```python
from build123d import *

# Parameters (mm, degrees)
RESSALTO_EXTRUS_O1_DEPTH = 6
CORTE_EXTRUS_O1_DEPTH    = 428.242320001
FILETE1_R                = 5
RESSALTO_EXTRUS_O3_DEPTH = 7
RESSALTO_EXTRUS_O4_DEPTH = 6
FILETE2_R                = 5
ESBO_O13_W               = 15
ESBO_O13_H               = 6
CORTE_EXTRUS_O2_DEPTH    = 428.242320001
ESBO_O15_W               = 15
ESBO_O15_H               = 6
CORTE_EXTRUS_O3_DEPTH    = 428.242320001


with BuildPart() as part:
    # Esboço2 → Ressalto-extrusão1 (new body)
    with BuildSketch(Plane.XY):
        Polygon((0, 0), (0, 400), (50, 400), (150, 20), (150, 0), align=None)
    extrude(amount=RESSALTO_EXTRUS_O1_DEPTH)

    # Esboço7 → Corte-extrusão1 (cut, through all)
    with BuildSketch(Plane(origin=(0, 0, 0), x_dir=(-1, 0, 0), z_dir=(0, 0, -1))):
        Polygon((-32.276413741, 20), (-32.276413741, 310), (-120, 20), align=None)
    extrude(amount=-CORTE_EXTRUS_O1_DEPTH, mode=Mode.SUBTRACT)

    # Filete1
    filete1_edges = [part.edges().sort_by_distance(p)[0] for p in [
        (32.276413741, 20, 3),
        (120, 20, 3),
        (32.276413741, 310, 3),
    ]]
    fillet(filete1_edges, radius=FILETE1_R)

    # Esboço11 → Ressalto-extrusão3 (add)
    with BuildSketch(Plane(origin=(0, 0, 0), x_dir=(-1, 0, 0), z_dir=(0, 0, -1))):
        Polygon((-85.790275479, 133.09182096), (-32.276413741, 133.09182096), (-32.276413741, 164.53133753), (-76.279974983, 164.53133753), align=None)
    extrude(amount=-RESSALTO_EXTRUS_O3_DEPTH)

    # Esboço12 → Ressalto-extrusão4 (add)
    with BuildSketch(Plane(origin=(0, 0, 0), x_dir=(-1, 0, 0), z_dir=(0, 0, -1))):
        Polygon((-85.790275479, 133.09182096), (-32.276413741, 29.65724659), (-27.594715127, 20), (-48.670406936, 20), (-94.468741252, 104.402215557), align=None)
    extrude(amount=-RESSALTO_EXTRUS_O4_DEPTH)

    # Filete2
    filete2_edges = [part.edges().sort_by_distance(p)[0] for p in [
        (32.276413741, 133.09182096, 3),
        (32.276413741, 164.53133753, 3),
        (85.790275479, 133.09182096, 3),
        (76.279974983, 164.53133753, 3),
        (94.468741252, 104.402215557, 3),
        (32.276413741, 29.65724659, 3),
        (48.670406936, 20, 3),
    ]]
    fillet(filete2_edges, radius=FILETE2_R)

    # Esboço13 → Corte-extrusão2 (cut, through all)
    with BuildSketch(Plane.XY.offset(6)):
        with Locations((7.5, 397)):
            Rectangle(ESBO_O13_W, ESBO_O13_H)
        with Locations((42.525660804, 397)):
            Rectangle(ESBO_O13_W, ESBO_O13_H)
    extrude(amount=-CORTE_EXTRUS_O2_DEPTH, mode=Mode.SUBTRACT)

    # Esboço15 → Corte-extrusão3 (cut, through all)
    with BuildSketch(Plane.XY.offset(6)):
        with Locations((7.5, 3)):
            Rectangle(ESBO_O15_W, ESBO_O15_H)
        with Locations((42.5, 3)):
            Rectangle(ESBO_O15_W, ESBO_O15_H)
        with Locations((142.5, 3)):
            Rectangle(ESBO_O15_W, ESBO_O15_H)
    extrude(amount=-CORTE_EXTRUS_O3_DEPTH, mode=Mode.SUBTRACT)


solid = part.part
```
Could you check a few things on this model? Use its own coordinates, in mm. A direction names the side the tool comes from. Coordinates: 2 decimals unless noted, no trailing zeros. Write each loop counter-clockwise with the first axis right and the second up, starting at its lowest first coordinate (ties: lowest second). Pieces come first, ordered by that corner, then holes. Notation, with made-up numbers: (83.25, -36) -> (138.25, -36) arc R17 cw to (138.25, -29) -> close; hole circle Ø9 at (-6, -33.75). An arc over 180 degrees is marked (long way). Write item = value, one per line. Start each with the question number.
(1) I want a section at D-D (x = 139.5). Please give me the cut outline in (y, z).
(2) I want a section at A-A (y = 259.5). Please give me the cut outline in (x, z).
(3) We'd pull the mould along X, two halves only. Please class faces 4 (the face through (99.313, 212.611, 2.958)), 5 (the face through (57, 158, 0)), 6 (the face through (59, 133.092, 3)): released by +X, released by -X, zero draft, split by the parting line, or undercut.
(4) Which directions (+Z, -Z, +X, -X, +Y, -Y) give clear straight access to the entire face, cutting with the end or side of a thin tool? Please do faces 1 (the face through (70.46, 60.16, 2.96)), 2 (the face through (80.97, 149.03, 6.49)), 3 (the face through (59, 149, 7)).
(5) Will these pins go through, and if not, where does the flat tip stop? pin 1 (3 mm diameter, centred on y = 395.5, z = 3.5, fed in from +X); pin 2 (3 mm diameter, centred on y = 1.5, z = 3, fed in from +X); pin 3 (5 mm diameter, centred on x = 76, y = 295, fed in from +Z).
(6) I want a section at C-C (y = 105.5). Please give me the cut outline in (x, z), plus the area to 3 significant figures.
(7) I want a section at B-B (z = 4). Give the number of separate pieces and of enclosed holes in the cut face, plus the area to 3 significant figures.
(8) I need wall thicknesses on line 1 (X direction, y = 59.5, z = 5.75); line 2 (Z direction, x = 63, y = 86); line 3 (X direction, y = 45, z = 2.25). Which ranges of each line are inside material? Lowest first, please. Write a range as [from, to].
Result set:
q1.outline = (6, 0) -> (59.9, 0) -> (59.9, 6) -> (6, 6) -> close
q2.outline = (0, 0) -> (32.28, 0) -> (32.28, 6) -> (0, 6) -> close; (47.55, 0) -> (86.97, 0) -> (86.97, 6) -> (47.55, 6) -> close
q3.face_4 = released by +X
q3.face_5 = zero draft
q3.face_6 = undercut
q4.face_1 = +Z, -Z
q4.face_2 = +Z, +X, +Y
q4.face_3 = +Z, +X, -X, +Y, -Y
q5.pin_1 = 51.58
q5.pin_2 = 135
q5.pin_3 = 6
q6.outline = (0, 0) -> (32.28, 0) -> (32.28, 6) -> (0, 6) -> close; (71.52, 0) -> (127.5, 0) -> (127.5, 6) -> (71.52, 6) -> close
q6.area = 530 mm2
q7.separate_pieces = 1
q7.enclosed_holes = 3
q7.area = 31,900 mm2
q8.line_1 = [0, 32.28], [47.72, 70.1], [108.05, 139.61]
q8.line_2 = [0, 6]
q8.line_3 = [0, 62.24], [112.44, 143.42]
